from build123d import *

# Parameters (mm, degrees)
F0_R     = 27.047238
F1_DEPTH = 5.4
F2_R     = 5.341981
F3_DEPTH = 25
F4_R     = 2.441964
F5_DEPTH = 48.8


with BuildPart() as f1:
    # F0 (on Front) → F1 (new body)
    with BuildSketch(Plane.XZ):
        Circle(F0_R)
    extrude(amount=F1_DEPTH)

    # F2 (on face) → F3 (join)
    with BuildSketch(Plane(origin=(0, 0, 0), x_dir=(-1, 0, 0), z_dir=(0, 1, 0))):
        Circle(F2_R)
    extrude(amount=F3_DEPTH)

    # F4 (on face) → F5 (cut, symmetric)
    with BuildSketch(Plane(origin=(0, 25, 0), x_dir=(-1, 0, 0), z_dir=(0, 1, 0))):
        Circle(F4_R)
    extrude(amount=F5_DEPTH, both=True, mode=Mode.SUBTRACT)


solid = f1.part
The model under review builds one solid part; all positions refer to its coordinate system, in mm. A direction names the side the tool comes from. Give positions to 0.01 mm unless a question says otherwise; leave off trailing zeros. Loops run counter-clockwise (first coordinate to the right, second up) from the corner with the lowest first, then second, coordinate; pieces in that order, holes last. Notation, with made-up numbers: (58.5, 87) -> (110.5, 87) arc R19 cw to (110.5, 94) -> close; hole circle Ø9 at (79.25, 8.5). An arc over 180 degrees is marked (long way). Answer as a JSON object with one key per item and string values. Group by question number.
Q1. Wall thickness on line 1 along Z through (x, y) = (0, 4); line 2 along Y through (x, z) = (-12, -13.5); line 3 along X through (y, z) = (21, -4): over which ranges is each line inside the solid? List them lowest first.
Q2. Take a section at A-A (z = 0). Write out the cut boundary in (x, y), plus the area to 3 significant figures.
Q3. Tool access review of faces 1 (the flat face through (6, -5.4, 0)), 2 (the cylindrical face through (0.695, 12.325, 5.297)): name each direction out of +Z, -Z, +X, -X, +Y, -Y from which nothing blocks a thin tool from reaching the whole face with its end or side.
Q4. Draft analysis for pull direction X (two halves, no side actions). For faces 3 (the cylindrical face through (1.938, 10.013, -1.486)), 4 (the cylindrical face through (24.985, -2.662, -10.359)), 5 (the flat face through (-2.3, 25, 1.3)), state which applies: pulls with the +X half, pulls with the -X half, needs draft (parallel to the pull), parting line crosses it, or undercut.
Q5. Take a section at C-C (y = 11.5). Write out the cut boundary in (x, z).
Q6. Insertion check: pin 1 (2 mm diameter, centred on x = 7.5, z = 4, fed in from +Y); pin 2 (3 mm diameter, centred on x = 3.5, y = 1, fed in from +Z); pin 3 (12 mm diameter, centred on y = 10, z = 8, fed in from +X). Each pin has a flat end and moves straight along its axis. Give the tip position at first contact, or say it passes through.
Q7. Take a section at B-B (x = 0). Write out the cut boundary in (y, z).
Q8. Take a section at D-D (x = -6.5). Write out the cut boundary in (y, z).
Answer below:
{
 "1": {"line 1": "z = -5.34 to -2.44, 2.44 to 5.34", "line 2": "y = -5.4 to 0", "line 3": "x = -3.54 to 3.54"},
 "2": {"outline": "(-27.05, -5.4) -> (-2.44, -5.4) -> (-2.44, 25) -> (-5.34, 25) -> (-5.34, 0) -> (-27.05, 0) -> close; (2.44, -5.4) -> (27.05, -5.4) -> (27.05, 0) -> (5.34, 0) -> (5.34, 25) -> (2.44, 25) -> close", "area": "411 mm2"},
 "3": {"face 1": "+Z, -Z, +X, -X, -Y", "face 2": "+Y"},
 "4": {"face 3": "undercut", "face 4": "parting line crosses it", "face 5": "needs draft"},
 "5": {"outline": "circle Ø10.68 at (0, 0); hole circle Ø4.88 at (0, 0)"},
 "6": {"pin 1": "stops at y = 0", "pin 2": "stops at z = 26.94", "pin 3": "stops at x = 4.95"},
 "7": {"outline": "(-5.4, -27.05) -> (0, -27.05) -> (0, -5.34) -> (25, -5.34) -> (25, -2.44) -> (-5.4, -2.44) -> close; (-5.4, 2.44) -> (25, 2.44) -> (25, 5.34) -> (0, 5.34) -> (0, 27.05) -> (-5.4, 27.05) -> close"},
 "8": {"outline": "(-5.4, -26.25) -> (0, -26.25) -> (0, 26.25) -> (-5.4, 26.25) -> close"}
}
